Geometry: see drawing. Coordinates: mm, zero at the bounding-box minimum. A direction names the side the tool comes from. Give positions to 0.01 mm unless a question says otherwise; leave off trailing zeros. Write each loop counter-clockwise with the first axis right and the second up, starting at its lowest first coordinate (ties: lowest second). Pieces come first, ordered by that corner, then holes. Notation, with made-up numbers: (77.5, 35) -> (129.5, 35) arc R34 ccw to (129.5, 71) -> close; hole circle Ø9 at (1.25, 0). An arc over 180 degrees is marked (long way). Use one line per item in the form item = value. Start each with the question number.
(1) Cut plane A-A, the plane z = 88.9. Output: boundary loops of the cut face in (x, y), and give its area (3 significant figures).
(2) Cut plane B-B, the plane x = 88.9. Output: boundary loops of the cut face in (y, z).
(3) Set-up query: the marked faces 1 and 2. Return all of +Z, -Z, +X, -X, +Y, -Y with unobstructed straight access to the full face (end or side cutting, diameter ignored); none if empty.
(4) First-contact query: P1, Ø8, axis at y = 15, z = 110, coming from the +X side; P2, Ø1, axis at x = 146, z = 42, coming from the +Y side; P3, Ø8, axis at x = 99, y = 10.5, coming from the -Z side. Flat tips, straight axial feed; report the tip coordinate or a pass-through.
(5) Draft query along Z for the marked faces 3, 4, 5 and 6. Return one class per face: pulls with the +Z half, pulls with the -Z half, needs draft (parallel to the pull), parting line crosses it, or undercut.
(6) Cut plane C-C, the plane y = 4.25. Count the separate pieces of the cut face and the enclosed holes in it, and give its area (3 significant figures).
(7) Material intervals for line 1 along Z through (x, y) = (55, 8) (1 decimal); line 2 along Z through (x, y) = (154, 12) (1 decimal); line 3 along Z through (x, y) = (168.5, 12.75) (1 decimal), sorted ascending. Write a range as from..to.
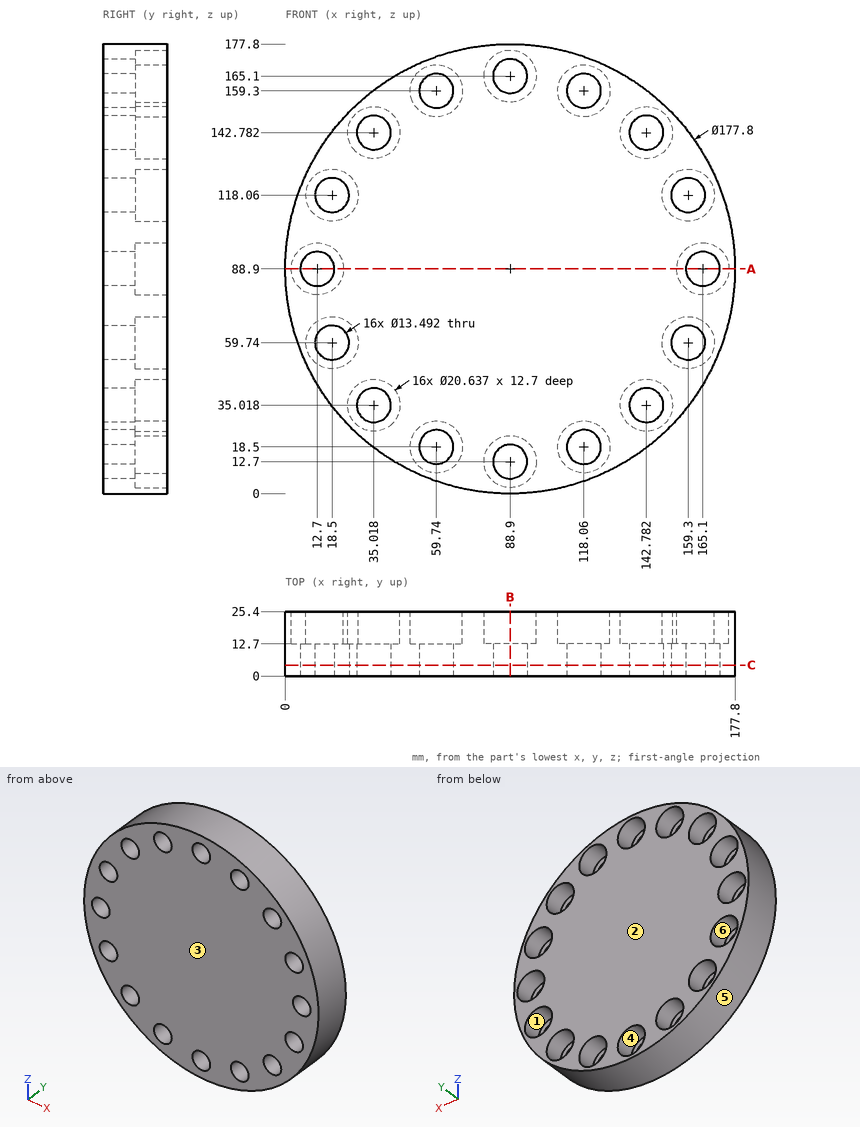
Geometry says:
q1.outline = (0, 0) -> (5.95, 0) -> (5.95, 12.7) -> (2.38, 12.7) -> (2.38, 25.4) -> (0, 25.4) -> close; (19.45, 0) -> (158.35, 0) -> (158.35, 12.7) -> (154.78, 12.7) -> (154.78, 25.4) -> (23.02, 25.4) -> (23.02, 12.7) -> (19.45, 12.7) -> close; (171.85, 0) -> (177.8, 0) -> (177.8, 25.4) -> (175.42, 25.4) -> (175.42, 12.7) -> (171.85, 12.7) -> close
q1.area = 3,650 mm^2
q2.outline = (0, 0) -> (25.4, 0) -> (25.4, 2.38) -> (12.7, 2.38) -> (12.7, 5.95) -> (0, 5.95) -> close; (0, 19.45) -> (12.7, 19.45) -> (12.7, 23.02) -> (25.4, 23.02) -> (25.4, 154.78) -> (12.7, 154.78) -> (12.7, 158.35) -> (0, 158.35) -> close; (0, 171.85) -> (12.7, 171.85) -> (12.7, 175.42) -> (25.4, 175.42) -> (25.4, 177.8) -> (0, 177.8) -> close
q3.face_1 = +Y
q3.face_2 = +Z, -Z, +X, -X, +Y
q4.P1 = 176.14
q4.P2 = 12.7
q4.P3 = 0.21
q5.face_3 = needs draft
q5.face_4 = undercut
q5.face_5 = parting line crosses it
q5.face_6 = undercut
q6.separate_pieces = 1
q6.enclosed_holes = 16
q6.area = 22,500 mm^2
q7.line_1 = 6.7..13.7, 23.3..154.5, 164.1..171.1
q7.line_2 = 28.4..55.6, 63.9..113.9, 122.2..149.4
q7.line_3 = 49.3..55.1, 64.4..79.2, 98.6..113.4, 122.7..128.5
